from build123d import *
from OCP.BRepFilletAPI import BRepFilletAPI_MakeChamfer

# Parameters (mm, degrees)
BOSS_EXTRUDE1_START = -0.7874
SKETCH3_R           = 19.05
SKETCH3_R_2         = 9.525
BOSS_EXTRUDE1_DEPTH = 1.5748
CHAMFER1_SIZE       = 0.15748
CHAMFER1_SIZE2      = 0.09092112
FILLET1_R           = 0.47244


with BuildPart() as part:
    # Sketch3 → Boss-Extrude1 (new body)
    with BuildSketch(Plane.XY.offset(BOSS_EXTRUDE1_START)):
        Circle(SKETCH3_R)
        Circle(SKETCH3_R_2, mode=Mode.SUBTRACT)
    extrude(amount=BOSS_EXTRUDE1_DEPTH)

    # Chamfer1: one chamfer whose edges measure the first distance from different faces: ONE call of the kernel's chamfer builder (chamfer() names one face for all edges)
    chamfer1_edges_1 = [part.edges().sort_by_distance(p)[0] for p in [
        (-19.05, 0, 0.7874),
    ]]
    chamfer1_side_1 = [part.faces().sort_by_distance(p)[0] for p in [
        (-19.05, 0, 0),
    ]]
    chamfer1_edges_2 = [part.edges().sort_by_distance(p)[0] for p in [
        (-9.525, 0, 0.7874),
    ]]
    chamfer1_side_2 = [part.faces().sort_by_distance(p)[0] for p in [
        (-9.525, 0, 0),
    ]]
    chamfer1 = BRepFilletAPI_MakeChamfer(part.part.solid().wrapped)
    for e in chamfer1_edges_1:
        chamfer1.Add(CHAMFER1_SIZE, CHAMFER1_SIZE2, e.wrapped, chamfer1_side_1[0].wrapped)  # the first distance lies on this face
    for e in chamfer1_edges_2:
        chamfer1.Add(CHAMFER1_SIZE, CHAMFER1_SIZE2, e.wrapped, chamfer1_side_2[0].wrapped)  # the first distance lies on this face
    add(Compound.cast(chamfer1.Shape()), mode=Mode.REPLACE)

    # Fillet1
    # the kernel refuses this fillet: 0.47244 mm, written as the material it takes off along each edge
    with BuildSketch(Plane(origin=(0, 0, 0.7874), x_dir=(1, 0, 0), z_dir=(0, -1, 0))) as fillet1_piece_1:
        with BuildLine():
            CenterArc((18.697864015, -0.47244), FILLET1_R, 41.810314896, 48.189685104)
            Line((18.697864015, 0), (18.697864015, 0.0094488))
            Line((18.697864015, 0.0094488), (18.95907888, 0.0094488))
            Line((18.95907888, 0.0094488), (18.96726178, 0.0047244))
            ThreePointArc((18.96726178, 0.0047244), (19.012722341, -0.0740156), (19.05704272, -0.1511808))
            Line((19.05704272, -0.1511808), (19.05, -0.15748))
        make_face()
    revolve(axis=Axis((0, 0, 0.7874), (0, 0, 1)), mode=Mode.SUBTRACT)
    with BuildSketch(Plane(origin=(0, 0, 0.7874), x_dir=(1, 0, 0), z_dir=(0, -1, 0))) as fillet1_piece_2:
        with BuildLine():
            CenterArc((9.877135985, -0.47244), FILLET1_R, 90, 48.189685104)
            Line((9.525, -0.15748), (9.51795728, -0.1511808))
            ThreePointArc((9.51795728, -0.1511808), (9.562277659, -0.0740156), (9.60773822, 0.0047244))
            Line((9.60773822, 0.0047244), (9.61592112, 0.0094488))
            Line((9.61592112, 0.0094488), (9.877135985, 0.0094488))
            Line((9.877135985, 0.0094488), (9.877135985, 0))
        make_face()
    revolve(axis=Axis((0, 0, 0.7874), (0, 0, 1)), mode=Mode.SUBTRACT)


solid = part.part
CAD build for the part. Positions are in the model's coordinates, mm. Give positions to 0.01 mm unless a question says otherwise; leave off trailing zeros. Order: outer loops, then holes, each group sorted by start corner. A loop starts at its lowest first (then second) coordinate and runs counter-clockwise, first axis right, second up. Notation, with made-up numbers: (44, 74.5) - (69, 74.5) arc R26 cw to (69, 103.5) - close; hole circle Ø6 at (-20, 36.5). An arc over 180 degrees is marked (long way). Write each question's results on one line, items separated by ' | '.
1. Pull direction Y, two halves, no side cores. Call faces 1 (the face through (4, 9, -0.787)), 2 (the face through (-7.559, -5.796, -0.089)), 3 (the face through (-15.12, -11.59, -0.09)): released by +Y, released by -Y, zero draft, split by the parting line, or undercut.
Calculated:
face 1: zero draft | face 2: undercut | face 3: split by the parting line
2. Saw through at A-A on y = 0. List the corners of the cut face in (x, z) (3 decimals), and give its area (3 significant figures).
Calculated:
outline: (-19.05, -0.787) - (-9.525, -0.787) - (-9.525, 0.63) arc R0.472 ccw to (-9.877, 0.787) - (-18.698, 0.787) arc R0.472 ccw to (-19.05, 0.63) - close; (9.525, -0.787) - (19.05, -0.787) - (19.05, 0.63) arc R0.472 ccw to (18.698, 0.787) - (9.877, 0.787) arc R0.472 ccw to (9.525, 0.63) - close | area: 29.9 mm2
3. Saw through at C-C on z = -0.35. List the corners of the cut face in (x, y) (3 decimals), and give its area (3 significant figures).
Calculated:
outline: circle Ø38.1 at (0, 0); hole circle Ø19.05 at (0, 0) | area: 855 mm2
4. Probe L1, parallel to Y at x = 0, z = -0.5 (3 decimals); L2, parallel to Y at x = 6, z = -0.05; L3, parallel to X at y = -5.5, z = -0.1. List the from-to ranges inside material, lowest first. Write a range as from..to.
Calculated:
L1: y = -19.05..-9.525, 9.525..19.05 | L2: y = -18.08..-7.4, 7.4..18.08 | L3: x = -18.24..-7.78, 7.78..18.24
